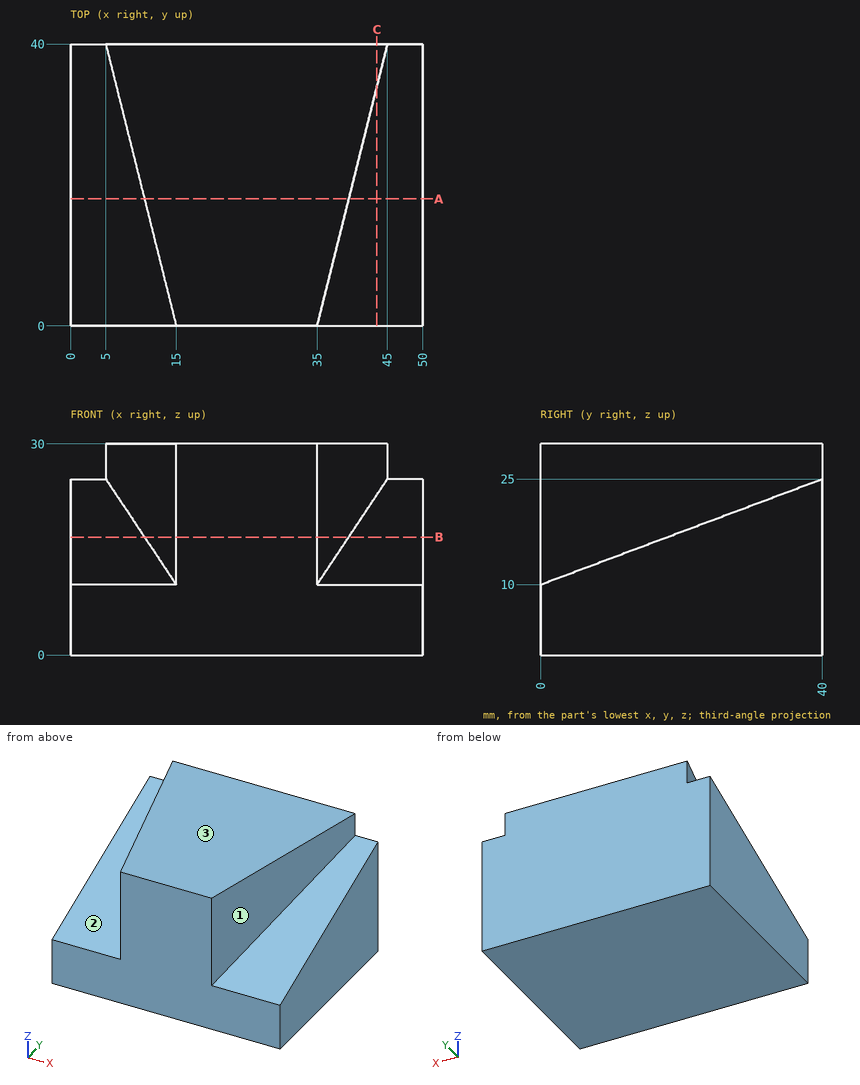
Here's the drawing with two shaded views (mm, measured from the low corner). I have some questions. A direction names the side the tool comes from. Coordinates: 2 decimals unless noted, no trailing zeros. Write each loop counter-clockwise with the first axis right and the second up, starting at its lowest first coordinate (ties: lowest second). Pieces come first, ordered by that corner, then holes. Notation, with made-up numbers: (89, -29.75) -> (99, -29.75) arc R27 ccw to (99, -13.75) -> close; hole circle Ø1 at (-21.75, 10). An arc over 180 degrees is marked (long way). Answer as CSV lines item,"result".
1) If I drill on line 1 (X direction, y = 17.5, z = 16.75) (3 decimals); line 2 (Z direction, x = 10, y = 18.5); line 3 (X direction, y = 22, z = 18.75), over which ranges is the centre line in solid material (lowest first)? Write a range as from..to.
Check result:
line 1,"10.625..39.375"
line 2,"0..16.94"
line 3,"9.5..40.5"
2) On a 3-axis mill with a long thin cutter (end or side, diameter ignored), from which of +Z, -Z, +X, -X, +Y, -Y can I reach the whole of each face in a straight line? I mean the marked faces 1, 2 and 3. Say none if no direction works.
Check result:
face 1,"+Z, +X, -Y"
face 2,"+Z, -X, -Y"
face 3,"+Z, +X, -X, +Y, -Y"
3) Will these pins go through, and if not, where does the flat tip stop? P1, Ø5, axis at y = 21.5, z = 18.5, coming from the -X side; P2, Ø6, axis at y = 14, z = 21, coming from the +X side.
Check result:
P1,"x = 0"
P2,"x = 39.25"
4) If we section it at B-B on z = 16.75: Please give me the cut outline in (x, y), then the cut area to 3 significant figures.
Check result:
outline,"(0, 18) -> (10.5, 18) -> (15, 0) -> (35, 0) -> (39.5, 18) -> (50, 18) -> (50, 40) -> (0, 40) -> close"
area,"1,540 mm²"
5) If we section it at C-C on x = 43.5: Please give me the cut outline in (y, z), then the cut area to 3 significant figures.
Check result:
outline,"(0, 0) -> (40, 0) -> (40, 30) -> (34, 30) -> (34, 22.75) -> (0, 10) -> close"
area,"737 mm²"
6) If we section it at A-A on y = 18: Please give me the cut outline in (x, z), then the cut area to 3 significant figures.
Check result:
outline,"(0, 0) -> (50, 0) -> (50, 16.75) -> (39.5, 16.75) -> (39.5, 30) -> (10.5, 30) -> (10.5, 16.75) -> (0, 16.75) -> close"
area,"1,220 mm²"
